Read the model definition and answer for the solid it produces. Units are mm, in the model's axes. Face numbers are marked on the shaded views. A direction names the side the tool comes from. Give positions to 0.01 mm unless a question says otherwise; leave off trailing zeros. Write each loop counter-clockwise with the first axis right and the second up, starting at its lowest first coordinate (ties: lowest second). Pieces come first, ordered by that corner, then holes. Notation, with made-up numbers: M 89.5,85 L 116.5,85 A13 cw 116.5,97 Z; hole C 78.25,-25.75 d9. An arc over 180 degrees is marked long. Put each result on its own line as item: value.
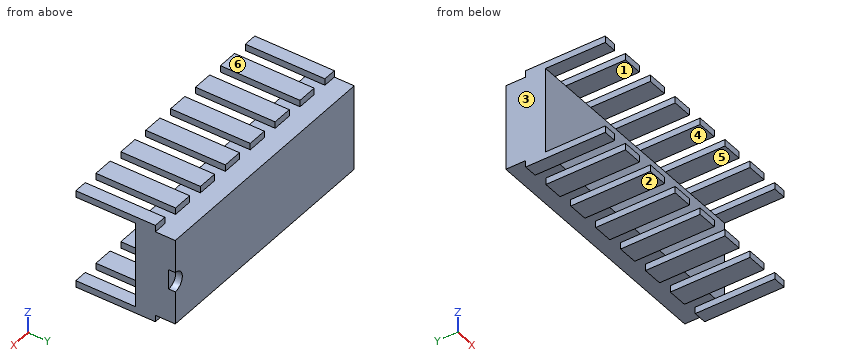
from build123d import *

# Parameters (mm, degrees)
EXTRUDE_1_DEPTH = 3
EXTRUDE_2_DEPTH = 2.5
EXTRUDE_START   = 1.5
SKETCH_1_4_W    = 1
SKETCH_1_4_H    = 0.5
SKETCH_1_4_W_2  = 1.5
EXTRUDE_3_DEPTH = 6


with BuildPart() as part:
    # Эскиз1 → Бобышка-Вытянуть1 (new body)
    with BuildSketch(Plane(origin=(0, 0, 0), x_dir=(1, 0, 0), z_dir=(0, 1, 0))):
        with BuildLine():
            Line((-8.5, 3.25), (-9.5, 3.25))
            Line((-9.5, 3.25), (-9.5, -3.25))
            Line((-9.5, -3.25), (-8.5, -3.25))
            Line((-8.5, -3.25), (-7.357142857, -3.25))
            Line((-7.357142857, -3.25), (-5.857142857, -3.25))
            Line((-5.857142857, -3.25), (-4.714285714, -3.25))
            Line((-4.714285714, -3.25), (-3.214285714, -3.25))
            Line((-3.214285714, -3.25), (-2.071428571, -3.25))
            Line((-2.071428571, -3.25), (-0.571428571, -3.25))
            Line((-0.571428571, -3.25), (0.571428571, -3.25))
            Line((0.571428571, -3.25), (2.071428571, -3.25))
            Line((2.071428571, -3.25), (3.214285714, -3.25))
            Line((3.214285714, -3.25), (4.714285714, -3.25))
            Line((4.714285714, -3.25), (5.857142857, -3.25))
            Line((5.857142857, -3.25), (7.357142857, -3.25))
            Line((7.357142857, -3.25), (8.5, -3.25))
            Line((8.5, -3.25), (9.5, -3.25))
            Line((9.5, -3.25), (9.5, -0.75))
            ThreePointArc((9.5, -0.75), (8.75, 0), (9.5, 0.75))
            Line((9.5, 0.75), (9.5, 3.25))
            Line((9.5, 3.25), (8.5, 3.25))
            Line((8.5, 3.25), (7.357142857, 3.25))
            Line((7.357142857, 3.25), (5.857142857, 3.25))
            Line((5.857142857, 3.25), (4.714285714, 3.25))
            Line((4.714285714, 3.25), (3.214285714, 3.25))
            Line((3.214285714, 3.25), (2.071428571, 3.25))
            Line((2.071428571, 3.25), (0.571428571, 3.25))
            Line((0.571428571, 3.25), (-0.571428571, 3.25))
            Line((-0.571428571, 3.25), (-2.071428571, 3.25))
            Line((-2.071428571, 3.25), (-3.214285714, 3.25))
            Line((-3.214285714, 3.25), (-4.714285714, 3.25))
            Line((-4.714285714, 3.25), (-5.857142857, 3.25))
            Line((-5.857142857, 3.25), (-7.357142857, 3.25))
            Line((-7.357142857, 3.25), (-8.5, 3.25))
        make_face()
    extrude(amount=EXTRUDE_1_DEPTH)

    # Эскиз1<3> → Бобышка-Вытянуть2 (add)
    with BuildSketch(Plane(origin=(0, 0, 0), x_dir=(1, 0, 0), z_dir=(0, 1, 0))):
        with BuildLine():
            Line((9.5, -0.75), (9.5, 0.75))
            ThreePointArc((9.5, 0.75), (8.75, 0), (9.5, -0.75))
        make_face()
    extrude(amount=EXTRUDE_2_DEPTH)

    # Эскиз1<4> → Бобышка-Вытянуть3 (add)
    with BuildSketch(Plane(origin=(0, 0, 0), x_dir=(1, 0, 0), z_dir=(0, 1, 0)).offset(EXTRUDE_START)):
        with Locations((-9, 3.5)):
            Rectangle(SKETCH_1_4_W, SKETCH_1_4_H)
        with Locations((-9, -3.5)):
            Rectangle(SKETCH_1_4_W, SKETCH_1_4_H)
        with Locations((-6.607142857, 3.5)):
            Rectangle(SKETCH_1_4_W_2, SKETCH_1_4_H)
        with Locations((-6.607142857, -3.5)):
            Rectangle(SKETCH_1_4_W_2, SKETCH_1_4_H)
        with Locations((-3.964285714, 3.5)):
            Rectangle(SKETCH_1_4_W_2, SKETCH_1_4_H)
        with Locations((-3.964285714, -3.5)):
            Rectangle(SKETCH_1_4_W_2, SKETCH_1_4_H)
        with Locations((-1.321428571, 3.5)):
            Rectangle(SKETCH_1_4_W_2, SKETCH_1_4_H)
        with Locations((-1.321428571, -3.5)):
            Rectangle(SKETCH_1_4_W_2, SKETCH_1_4_H)
        with Locations((1.321428571, 3.5)):
            Rectangle(SKETCH_1_4_W_2, SKETCH_1_4_H)
        with Locations((1.321428571, -3.5)):
            Rectangle(SKETCH_1_4_W_2, SKETCH_1_4_H)
        with Locations((3.964285714, 3.5)):
            Rectangle(SKETCH_1_4_W_2, SKETCH_1_4_H)
        with Locations((3.964285714, -3.5)):
            Rectangle(SKETCH_1_4_W_2, SKETCH_1_4_H)
        with Locations((6.607142857, 3.5)):
            Rectangle(SKETCH_1_4_W_2, SKETCH_1_4_H)
        with Locations((6.607142857, -3.5)):
            Rectangle(SKETCH_1_4_W_2, SKETCH_1_4_H)
        with Locations((9, 3.5)):
            Rectangle(SKETCH_1_4_W, SKETCH_1_4_H)
        with Locations((9, -3.5)):
            Rectangle(SKETCH_1_4_W, SKETCH_1_4_H)
    extrude(amount=-EXTRUDE_3_DEPTH)


solid = part.part
(1) Given pin 1 Ø1 at (y, z) = (-1, 1) entering from -X; pin 2 Ø1 at (x, z) = (-6.5, -1) entering from -Y, each flat-ended and moving along its own axis, determine where each tip first touches the part or whether it passes through.
Result:
pin 1: passes through
pin 2: stops at y = 0
(2) Section A-A on y = -2.5 is taken. Give the number of separate pieces and of enclosed holes in the cut face, and give its area (3 significant figures).
Result:
separate pieces: 16
enclosed holes: 0
area: 11.0 mm²
(3) Section B-B on x = -1.25 is taken. Determine the outline of the cut face in (y, z), and give its area (3 significant figures).
Result:
outline: M -4.5,-3.75 L 1.5,-3.75 L 1.5,-3.25 L 3,-3.25 L 3,3.25 L 1.5,3.25 L 1.5,3.75 L -4.5,3.75 L -4.5,3.25 L 0,3.25 L 0,-3.25 L -4.5,-3.25 Z
area: 25.5 mm²
(4) For a pull along Z with two mould halves and no side action, classify the marked faces 1, 2, 3 and 4 as +Z half, -Z half, draft (parallel to the pull), parting line (faces both ways), or undercut.
Result:
face 1: undercut
face 2: -Z half
face 3: draft
face 4: undercut
(5) Which of the six approach directions +Z, -Z, +X, -X, +Y, -Y give full straight-line access (tool end or side, diameter ignored) to the marked faces 5 and 6?
Result:
face 5: +X, -X, -Y
face 6: +Z, +X, -X, +Y, -Y
(6) Straight lines are drawn through the part: line 1 along Z through (x, y) = (-4.5, -3); line 2 along Y through (x, z) = (-6, -0.25); line 3 along Y through (x, z) = (3.25, -3.5). For each, find the intervals that lie inside material, in ascending order. Write a range as from..to.
Result:
line 1: z = -3.75..-3.25, 3.25..3.75
line 2: y = 0..3
line 3: y = -4.5..1.5
(7) Section C-C on z = 0 is taken. Determine the outline of the cut face in (x, y), and give its area (3 significant figures).
Result:
outline: M -9.5,0 L 9.5,0 L 9.5,2.5 L 8.75,2.5 L 8.75,3 L -9.5,3 Z
area: 56.6 mm²
(8) Section D-D on x = 5 is taken. Determine the outline of the cut face in (y, z), and give its area (3 significant figures).
Result:
outline: M 0,-3.25 L 3,-3.25 L 3,3.25 L 0,3.25 Z
area: 19.5 mm²
